Read the model definition and answer for the solid it produces. Units are mm, in the model's axes. A direction names the side the tool comes from. Give positions to 0.01 mm unless a question says otherwise; leave off trailing zeros. Loops run counter-clockwise (first coordinate to the right, second up) from the corner with the lowest first, then second, coordinate; pieces in that order, holes last. Notation, with made-up numbers: (75, 12) -> (79, 12) arc R36 ccw to (79, 51) -> close; hole circle Ø5 at (28, 55.5). An arc over 180 degrees is marked (long way). Answer as CSV lines item,"result". Start each with the question number.
Autodesk Inventor part; units mm, degrees
ref_plane "YZ Plane" through (0, 0, 0) normal (1, 0, 0) x (0, 1, 0)
ref_plane "XZ Plane" through (0, 0, 0) normal (0, 1, 0) x (-1, 0, 0)
ref_plane "XY Plane" through (0, 0, 0) normal (0, 0, 1) x (1, 0, 0)
sketch "Sketch1" plane through (0, 0, 0) normal (0, 1, 0) x (-1, 0, 0)
  line L0 (30.8368, 11.4286) -> (-9.1632, 11.4286)
  line L1 (-9.1632, 11.4286) -> (-9.1632, -28.5714)
  line L2 (-9.1632, -28.5714) -> (30.8368, -28.5714)
  line L3 (30.8368, -28.5714) -> (30.8368, 11.4286)
  point P0 (0, 0)
  dimension "d0" = 40
  dimension "d1" = 40
extrude "Extrusion1" add sketch "Sketch1" along normal blind 5
sketch "Sketch7" plane through (9.1632, 0, -28.5714) normal (1, 0, 0) x (0, 0, -1)
  point P0 (-28.5714, 0)
sketch "Sketch8" plane through (0, 0, 0) normal (0, -1, 0) x (1, 0, 0)
  point P0 (0, 0)
sketch "Sketch11" plane through (0, 5, 0) normal (0, 1, 0) x (1, 0, 0)
  line L0 (9.1632, -11.4286) -> (9.1632, 28.5714)
  line L1 (9.1632, 18.5714) -> (-0.8368, 18.5714)
  line L2 (-0.8368, 18.5714) -> (-0.8368, -1.4286)
  line L3 (-0.8368, -1.4286) -> (9.1632, -1.4286)
  line L4 (9.1632, -1.4286) -> (9.1632, 18.5714)
  line L5 (-30.8368, -11.4286) -> (9.1632, -11.4286)
  point P0 (0, 0)
  dimension "d29" = 10
  dimension "d30" = 20
  dimension "d31" = 10
extrude "Extrusion7" add sketch "Sketch11" along normal blind 5
sketch "Sketch12" plane through (0, 10, 0) normal (0, 1, 0) x (1, 0, 0)
  line L0 (9.1632, -1.4286) -> (9.1632, 18.5714)
  line L1 (3.175, 13.5714) -> (9.1632, 13.5714)
  line L2 (9.1632, 13.5714) -> (9.1632, 3.5714)
  line L3 (9.1632, 3.5714) -> (3.175, 3.5714)
  line L4 (3.175, 3.5714) -> (3.175, 13.5714)
  line L5 (9.1632, 18.5714) -> (-0.8368, 18.5714)
  point P0 (0, 0)
  dimension "d34" = 10
  dimension "d35" = 5
extrude "Extrusion8" add sketch "Sketch12" along normal blind 2.5
sketch "Sketch13" plane through (9.1632, 0, 11.4286) normal (1, 0, 0) x (0, 0, -1)
  line L0 (25, 12.5) -> (15, 12.5)
  line L1 (30, 10) -> (10, 10)
  line L2 (18, 12.5) -> (22, 12.5)
  line L3 (22, 12.5) -> (22, 10)
  line L4 (22, 10) -> (18, 10)
  line L5 (18, 10) -> (18, 12.5)
  line L6 (15, 10) -> (15, 12.5)
  point P0 (11.4286, 0)
  dimension "d38" = 4
  dimension "d39" = 3
extrude "Extrusion9" add sketch "Sketch13" along normal blind 4 contours L3 L1 L5 L0
sketch "Sketch14" plane through (0, 0, 0) normal (0, -1, 0) x (1, 0, 0)
  line L0 (4.1632, 6.4286) -> (-25.8368, 6.4286)
  line L1 (-25.8368, 6.4286) -> (-25.8368, -23.5714)
  line L2 (-25.8368, -23.5714) -> (4.1632, -23.5714)
  line L3 (4.1632, -23.5714) -> (4.1632, 6.4286)
  line L4 (9.1632, 11.4286) -> (9.1632, -28.5714)
  line L5 (9.1632, -28.5714) -> (-30.8368, -28.5714)
  point P0 (0, 0)
  dimension "d42" = 30
  dimension "d43" = 30
  dimension "d44" = 5
  dimension "d45" = 5
extrude "Extrusion10" add sketch "Sketch14" along normal blind 4
sketch "Sketch15" plane through (13.1632, 0, 11.4286) normal (1, 0, 0) x (0, 0, -1)
  line L0 (25, 12.5) -> (15, 12.5)
  line L1 (18.0261, 12.5) -> (22.0261, 12.5)
  line L2 (22.0261, 12.5) -> (22.0261, -15.875)
  line L3 (22.0261, -15.875) -> (18.0261, -15.875)
  line L4 (18.0261, -15.875) -> (18.0261, 12.5)
  point P0 (11.4286, 0)
  dimension "d48" = 4
extrude "Extrusion11" add sketch "Sketch15" along normal blind 4
sketch "Sketch30" plane through (13.1632, -15.875, -6.5975) normal (0, 0, 1) x (1, 0, 0)
  point P0 (-13.1632, 15.875)
sketch "Sketch31" plane through (17.1632, 0, 11.4286) normal (1, 0, 0) x (0, 0, -1)
  line L0 (18.0261, 10) -> (18.0261, -15.875)
  line L1 (22.0261, -15.875) -> (22.0261, 12.5)
  line L2 (18.0261, -15.875) -> (22.0261, -15.875)
  line L3 (22.0261, -15.875) -> (22.0261, -13.875)
  line L4 (22.0261, -13.875) -> (18.0261, -13.875)
  line L5 (18.0261, -13.875) -> (18.0261, -15.875)
  line L6 (18.0261, 12.5) -> (22.0261, 12.5)
  line L7 (22.0261, 12.5) -> (22.0261, -15.875)
  line L8 (22.0261, -15.875) -> (18.0261, -15.875)
  line L9 (18.0261, -15.875) -> (18.0261, 12.5)
  point P0 (11.4286, 0)
  dimension "d75" = 2
extrude "Extrusion21" cut sketch "Sketch31" against normal blind 4 contours L9 L6 L1 L4 L0
sketch "Sketch32" plane through (17.1632, 0, 11.4286) normal (1, 0, 0) x (0, 0, -1)
  line L0 (15.875, -11.1125) -> (23.8125, -11.1125)
  line L1 (23.8125, -11.1125) -> (23.8125, -20.6375)
  line L2 (23.8125, -20.6375) -> (15.875, -20.6375)
  line L3 (15.875, -20.6375) -> (15.875, -11.1125)
  point P0 (11.4286, 0)
extrude "Extrusion22" cut sketch "Sketch32" against normal blind 4
sketch "Sketch33" plane through (13.1632, 0, 11.4286) normal (1, 0, 0) x (0, 0, -1)
  line L0 (25, 12.5) -> (15, 12.5)
  line L1 (5, 0) -> (35, 0)
  line L2 (18, 12.5) -> (22, 12.5)
  line L3 (22, 12.5) -> (22, 0)
  line L4 (22, 0) -> (18, 0)
  line L5 (18, 0) -> (18, 12.5)
  line L6 (18, 12.5) -> (18, 10)
  point P0 (11.4286, 0)
  dimension "d80" = 4
  dimension "d81" = 0
extrude "Extrusion23" add sketch "Sketch33" along normal blind 4
sketch "Sketch34" plane through (17.1632, 0, 11.4286) normal (1, 0, 0) x (0, 0, -1)
  line L0 (5, 0) -> (35, 0)
  line L1 (22, 0) -> (22, 10)
  line L2 (18, 0) -> (22, 0)
  line L3 (22, 0) -> (22, 2)
  line L4 (22, 2) -> (18, 2)
  line L5 (18, 2) -> (18, 0)
  line L6 (18, 12.5) -> (18, 0)
  point P0 (11.4286, 0)
  dimension "d84" = 2
  dimension "d85" = 0
extrude "Extrusion24" add sketch "Sketch34" along normal blind 2
sketch "Sketch35" plane through (17.1632, 2, -6.5714) normal (0, 1, 0) x (1, 0, 0)
  point P0 (-17.1632, -6.5714)
sketch "Sketch36" plane through (19.1632, 0, 11.4286) normal (1, 0, 0) x (0, 0, -1)
  line L0 (22, 0) -> (22, 10)
  line L1 (22, 2) -> (18, 2)
  line L2 (18, 2) -> (18, 0)
  line L3 (18, 0) -> (22, 0)
  line L4 (22, 0) -> (22, 2)
  point P0 (11.4286, 0)
  dimension "d88" = 4
  dimension "d89" = 2
extrude "Extrusion25" add sketch "Sketch36" along normal blind 2
sketch "Sketch37" plane through (17.1632, 2, -6.5714) normal (0, 1, 0) x (1, 0, 0)
  line L0 (2, 3.175) -> (4, 3.175)
  line L1 (4, 3.175) -> (4, 1.175)
  line L2 (4, 1.175) -> (2, 1.175)
  line L3 (2, 1.175) -> (2, 3.175)
  line L4 (4, 4) -> (4, 0)
  point P0 (-17.1632, -6.5714)
  dimension "d92" = 2
  dimension "d93" = 2
  dimension "d94" = 0
extrude "Extrusion26" add sketch "Sketch37" along normal blind 18
sketch "Sketch38" plane through (17.1632, 20, -6.5714) normal (0, 1, 0) x (1, 0, 0)
  line L0 (-2, 3.175) -> (8, 3.175)
  line L1 (8, 3.175) -> (8, 1.175)
  line L2 (8, 1.175) -> (-2, 1.175)
  line L3 (-2, 1.175) -> (-2, 3.175)
  line L4 (4, 3.175) -> (2, 3.175)
  line L5 (4, 1.175) -> (4, 3.175)
  line L6 (2, 3.175) -> (2, 1.175)
  point P0 (-17.1632, -6.5714)
  dimension "d97" = 2
  dimension "d98" = 0
  dimension "d99" = 4
  dimension "d100" = 4
extrude "Extrusion27" add sketch "Sketch38" along normal blind 4
fillet "Fillet1" radius 1 4 edges at (21.1632, 11, -9.7464) (19.1632, 11, -9.7464) (19.1632, 11, -7.7464) (21.1632, 11, -7.7464)
sketch "Sketch40" plane through (15.1632, 24, -7.7464) normal (0, 0, 1) x (1, 0, 0)
  circle A0 centre (5.0665, -1.7928) radius 0.3
  point P0 (-15.1632, -24)
  dimension "d110" = 0.6
extrude "Extrusion29" cut sketch "Sketch40" against normal blind 100
sketch "Sketch41" plane through (15.1632, 24, -7.7464) normal (0, 0, 1) x (1, 0, 0)
  circle A0 centre (5.0665, -1.7928) radius 0.3
  circle A1 centre (5.0665, -1.7928) radius 0.3
  point P0 (-15.1632, -24)
sketch "Sketch42" plane through (0, -4, 0) normal (0, -1, 0) x (1, 0, 0)
  line L0 (4.1632, 6.4286) -> (4.1632, -23.5714)
  line L1 (-25.8368, 6.4286) -> (4.1632, 6.4286)
  line L2 (4.1632, -23.5714) -> (-25.8368, -23.5714)
  line L3 (-25.8368, -23.5714) -> (-25.8368, 6.4286)
  line L4 (-25.8368, 6.4286) -> (4.1632, 6.4286)
  line L5 (4.1632, 6.4286) -> (4.1632, -23.5714)
  point P0 (0, 0)
extrude "Extrusion30" add sketch "Sketch42" along normal blind 10
sketch "Sketch43" plane through (0, 12.5, 0) normal (0, 1, 0) x (1, 0, 0)
  line L0 (4.973, 9.5849) -> (6.6857, 10.5243)
  line L1 (6.6857, 10.5243) -> (8.3555, 9.5108)
  line L2 (8.3555, 9.5108) -> (8.3127, 7.5579)
  line L3 (8.3127, 7.5579) -> (6.6, 6.6185)
  line L4 (6.6, 6.6185) -> (4.9302, 7.632)
  line L5 (4.9302, 7.632) -> (4.973, 9.5849)
  point P0 (0, 0)
  point P1 (6.6429, 8.5714)
extrude "Extrusion31" add sketch "Sketch43" along normal blind 1
sketch "Sketch44" plane through (0, 0, 0) normal (0, -1, 0) x (1, 0, 0)
  circle A0 centre (6.6857, -8.642) radius 1.5
  point P0 (0, 0)
  dimension "d117" = 3
extrude "Extrusion32" add sketch "Sketch44" along normal blind 1
sketch "Sketch45" plane through (4.1632, 0, -23.5714) normal (0, 0, -1) x (-1, 0, 0)
  line L0 (30, -14) -> (0, -14)
  line L1 (30, 0) -> (30, -14)
  line L2 (0, -14) -> (30, -14)
  line L3 (30, -14) -> (30, -5.1197)
  line L4 (30, -5.1197) -> (0, -5.1197)
  line L5 (0, -5.1197) -> (0, -14)
  point P0 (4.1632, 0)
extrude "Extrusion33" cut sketch "Sketch45" against normal blind 100
sketch "Sketch46" plane through (-25.8368, -5.1197, -23.5714) normal (0, -1, 0) x (1, 0, 0)
  point P0 (25.8368, 23.5714)
sketch "Sketch47" plane through (9.1632, 0, 11.4286) normal (1, 0, 0) x (0, 0, -1)
  line L0 (35, -5.1197) -> (5, -5.1197)
  line L1 (40, 5) -> (0, 5)
  line L2 (35, -5.1197) -> (0, -5.1197)
  line L3 (0, -5.1197) -> (0, 5)
  line L4 (0, 5) -> (35, 5)
  line L5 (30, 5) -> (40, 5)
  line L6 (35, 5) -> (40, 5)
  line L7 (40, 0) -> (40, 5)
  line L8 (40, 5) -> (40, -5.1197)
  line L9 (40, -5.1197) -> (33.3375, -5.1197)
  point P0 (11.4286, 0)
  point P1 (5, -5.1197)
extrude "Extrusion34" cut sketch "Sketch47" against normal blind 4
properties part number "upper plate"
(1) Find section B-B on x = 18. Write down the section's boundary in (y, z).
(2) Find section D-D on x = -8. Write down the section's boundary in (y, z), then the cut area to 3 significant figures.
(3) Each of these flat-tipped pins is pushed along its axis until it touches: P1, Ø10, axis at y = 4, z = -7.5, coming from the +X side; P2, Ø0.8, axis at y = 11, z = -8.5, coming from the -X side (3 decimals); P3, Ø1, axis at x = 6.5, z = -9, coming from the +Y side. Where does it stop, or does it pass through?
(4) Find section C-C on z = -12.5. Write down the section's boundary in (x, y) (3 decimals), then the cut area to 3 significant figures.
(5) A tool of negligible diameter and unlimited length cuts with its end or side. For faces 1 (the face through (21, 22, -9.746)), 2 (the face through (4, 7, 1.429)), 3 (the face through (-13, 2, -28.571)), 4 (the face through (3.175, 11, -9)), 5 (the face through (-11, -3, -23.571)), from which of +Z, -Z, +X, -X, +Y, -Y can it reach the whole face along a straight path? Write none if from no direction.
(6) Find section A-A on y = 4. Give the number of separate pieces and of enclosed holes in the cut face, then the cut area to 3 significant figures.
(7) Find the intervals of material crossed by line 1 along Y through (x, z) = (1.5, 2); line 2 along Z through (x, y) = (-5, -0.5); line 3 along X through (y, z) = (0.25, -5.5), in increasing order. Write a range as from..to.
(8) The mould has two halves that part along X. Classify faces 6 (the face through (19, 2, -9)), 7 (the face through (17, 0, -9)), 8 (the face through (15.163, 22, -9)): pulls with the +X half, pulls with the -X half, needs draft (parallel to the pull), parting line crosses it, or undercut.
Answer block:
1,outline,"(0, -10.57) -> (2, -10.57) -> (2, -6.57) -> (0, -6.57) -> close; (20, -9.75) -> (24, -9.75) -> (24, -7.75) -> (20, -7.75) -> close"
2,outline,"(-5.12, -23.57) -> (0, -23.57) -> (0, -28.57) -> (5, -28.57) -> (5, 11.43) -> (0, 11.43) -> (0, 6.43) -> (-5.12, 6.43) -> close"
2,area,"354 mm2"
3,P1,"stops at x = 21.16"
3,P2,"stops at x = 3.175"
3,P3,"stops at y = 13.5"
4,outline,"(-30.837, 0) -> (-25.837, 0) -> (-25.837, -5.12) -> (4.163, -5.12) -> (4.163, 0) -> (5.163, 0) -> (5.163, 5) -> (9.163, 5) -> (9.163, 12.5) -> (3.175, 12.5) -> (3.175, 10) -> (-0.837, 10) -> (-0.837, 5) -> (-30.837, 5) -> close"
4,area,"399 mm2"
5,face 1,"-Z, +X, -X, +Y"
5,face 2,"+Z, +X, -X, +Y"
5,face 3,"-Z, +X, -X, +Y, -Y"
5,face 4,"+Z, -Z, -X, +Y"
5,face 5,"-Z, +X, -X, -Y"
6,separate pieces,"3"
6,enclosed holes,"0"
6,area,"1,460 mm2"
7,line 1,"y = -5.12..5"
7,line 2,"z = -23.57..6.43"
7,line 3,"x = -30.84..5.16"
8,face 6,"undercut"
8,face 7,"needs draft"
8,face 8,"pulls with the -X half"
